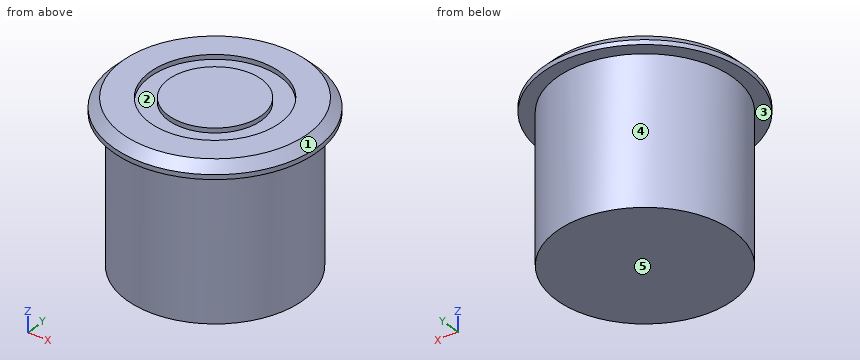
from build123d import *

# Parameters (mm, degrees)
F2_R     = 7
F2_R_2   = 5
F3_DEPTH = 0.5


with BuildPart() as f1:
    # F0 (on Right) → F1 (revolve)
    with BuildSketch(Plane.YZ):
        Polygon((0, 17.2), (0, 0), (9.5, 0), (9.5, 15.7), (11, 15.7), (11, 16.2), (10, 17.2), align=None)
    revolve(axis=Axis((0, 0, 8.6), (0, 0, 1)))

    # F2 (on face) → F3 (cut)
    with BuildSketch(Plane.XY.offset(17.2)):
        Circle(F2_R)
        Circle(F2_R_2, mode=Mode.SUBTRACT)
    extrude(amount=-F3_DEPTH, mode=Mode.SUBTRACT)


solid = f1.part
Here's how the part is built. I have some questions about the finished solid (model axes, mm). Face numbers are marked on the shaded views. A direction names the side the tool comes from. Give positions to 0.01 mm unless a question says otherwise; leave off trailing zeros. Loops run counter-clockwise (first coordinate to the right, second up) from the corner with the lowest first, then second, coordinate; pieces in that order, holes last. Notation, with made-up numbers: (35.5, 29) -> (73.5, 29) arc R24 ccw to (73.5, 56) -> close; hole circle Ø3 at (47.5, 31). An arc over 180 degrees is marked (long way). Answer as a JSON object with one key per item and string values. Group by question number.
Item 1: On a 3-axis mill with a long thin cutter (end or side, diameter ignored), from which of +Z, -Z, +X, -X, +Y, -Y can I reach the whole of each face in a straight line? I mean the marked faces 4 and 5. Say none if no direction works.
Item 2: I need wall thicknesses on L1, parallel to Y at x = 0, z = 17.05; L2, parallel to Y at x = 0, z = 16.85; L3, parallel to Z at x = 5, y = 1.75. Which ranges of each line are inside material? Lowest first, please.
Item 3: Will these pins go through, and if not, where does the flat tip stop? pin 1 (2 mm diameter, centred on x = -4.5, z = 12.5, fed in from -Y); pin 2 (6 mm diameter, centred on x = -4.5, z = 11, fed in from -Y); pin 3 (5 mm diameter, centred on y = -2.5, z = 9, fed in from -X).
Item 4: Imagine slicing it at A-A on y = 0. Write out the boundary of the cut face in (x, z).
Item 5: Imagine slicing it at C-C on z = 13. Write out the boundary of the cut face in (x, y), then the cut area to 3 significant figures.
Item 6: Thinking about a two-plate mould opening in X: for the marked faces 1, 2 and 3, which applies, pulls with the +X half, pulls with the -X half, needs draft (parallel to the pull), parting line crosses it, or undercut?
Answer list:
{
 "1": {"face 4": "-Z", "face 5": "-Z, +X, -X, +Y, -Y"},
 "2": {"L1": "y = -10.15 to -7, -5 to 5, 7 to 10.15", "L2": "y = -10.35 to -7, -5 to 5, 7 to 10.35", "L3": "z = 0 to 16.7"},
 "3": {"pin 1": "stops at y = -8.83", "pin 2": "stops at y = -9.38", "pin 3": "stops at x = -9.5"},
 "4": {"outline": "(-11, 15.7) -> (-9.5, 15.7) -> (-9.5, 0) -> (9.5, 0) -> (9.5, 15.7) -> (11, 15.7) -> (11, 16.2) -> (10, 17.2) -> (7, 17.2) -> (7, 16.7) -> (5, 16.7) -> (5, 17.2) -> (-5, 17.2) -> (-5, 16.7) -> (-7, 16.7) -> (-7, 17.2) -> (-10, 17.2) -> (-11, 16.2) -> close"},
 "5": {"outline": "circle Ø19 at (0, 0)", "area": "284 mm2"},
 "6": {"face 1": "parting line crosses it", "face 2": "undercut", "face 3": "needs draft"}
}
